Read the model definition and answer for the solid it produces. Units are mm, in the model's axes. A direction names the side the tool comes from. Coordinates: 2 decimals unless noted, no trailing zeros. Write each loop counter-clockwise with the first axis right and the second up, starting at its lowest first coordinate (ties: lowest second). Pieces come first, ordered by that corner, then holes. Notation, with made-up numbers: (-36, 47) -> (-25, 47) arc R14 ccw to (-25, 70) -> close; hole circle Ø10 at (24, 68.25). An arc over 180 degrees is marked (long way). One line per item, written item: value. Start each with the question number.
1. Given P1, Ø10, axis at x = 24, y = 45, coming from the -Z side; P2, Ø0.6, axis at y = 44, z = 1, coming from the +X side; P3, Ø1, axis at y = 37.5, z = 1, coming from the -X side; P4, Ø0.7, axis at y = 53.5, z = 0.5, coming from the +X side, each flat-ended and moving along its own axis, determine where each tip first touches the part or whether it passes through.
2. Find section A-A, the plane y = 35.5. Write down the section's boundary in (x, z).
3. Consider line 1 along X through (y, z) = (54.5, 1.95); line 2 along X through (y, z) = (43.5, 0.45); line 3 along Y through (x, z) = (15.5, 1.6). Determine where each line is inside the solid, lowest interval first.
4. For faces 1 (the flat face through (28.1, 57.08, 0.99)), 2 (the flat face through (41.827, 49.47, 0.986)), 3 (the flat face through (10.378, 39, 1)), determine the directions among +Z, -Z, +X, -X, +Y, -Y from which every point of the face is accessible in a straight line to the end or side of a thin tool.
5. Find section B-B, the plane x = 29. Write down the section's boundary in (y, z).
```python
from build123d import *

# Parameters (mm, degrees)
F1_DEPTH = 2


with BuildPart() as f1:
    # F0 (on Top) → F1 (new body)
    with BuildSketch(Plane.XY):
        Polygon((10.316424, 46.21381), (10.378422, 45.792866), (10.378422, 32.24406), (10.922515, 31.239605), (11.388969, 30.782871), (12.3236, 30.607224), (13.063584, 30.607224), (13.980744, 31.123197), (14.411193, 31.909108), (14.195969, 45.771692), (14.505405, 46.336659), (14.951889, 46.75483), (15.547823, 46.764082), (16.267732, 46.618171), (16.767925, 46.196714), (16.955901, 45.625031), (17.061751, 38.807264), (17.342532, 38.290832), (17.816337, 37.93142), (18.39029, 37.777532), (19.1046, 37.788622), (19.633163, 38.07852), (19.958686, 38.672859), (20.130083, 39.338022), (20.130083, 45.869723), (20.224372, 46.235643), (20.517316, 46.503272), (21.081642, 46.512033), (39.306525, 46.794985), (39.82532, 47.116615), (40.338621, 47.479954), (41.258305, 48.273247), (41.635639, 48.962181), (42.02386, 49.992487), (42.008081, 51.008835), (41.635639, 51.823597), (40.777957, 52.81793), (39.679653, 53.419479), (38.45059, 53.736179), (37.345576, 53.719023), (36.693033, 53.5032), (35.996381, 52.902289), (35.486977, 52.462892), (35.121937, 52.148019), (34.468539, 52.243274), (33.846248, 52.497253), (33.542935, 53.056076), (33.542935, 53.990863), (33.238664, 54.682236), (32.856002, 55.402562), (32.352884, 55.98584), (31.721991, 56.476444), (30.923305, 56.91389), (30.231845, 57.161622), (29.377455, 57.263315), (28.54972, 57.161622), (27.647492, 56.998174), (27.101057, 56.685288), (26.424225, 56.101473), (25.806281, 55.568452), (25.401196, 55.0007), (25.182293, 54.601029), (24.914882, 54.112791), (24.691492, 53.920102), (24.348679, 53.857998), (23.43077, 53.843747), (23.063278, 54.269789), (22.938367, 54.959297), (22.745963, 55.637598), (22.354444, 56.271017), (21.897662, 56.998174), (21.295404, 57.541236), (20.676884, 57.880004), (19.87285, 58.320378), (18.866845, 58.30476), (17.419982, 58.282296), (16.487831, 58.031149), (15.852839, 57.576239), (15.281766, 57.083648), (14.737288, 56.613998), (14.181019, 55.884421), (13.927415, 55.262856), (13.732859, 54.507815), (13.479641, 54.045492), (13.071425, 53.935507), (12.569794, 53.845812), (12.017341, 54.134376), (11.315221, 54.545794), (9.885113, 54.914299), (8.924496, 54.899385), (7.908149, 54.625553), (7.127685, 54.270785), (6.658861, 53.866391), (6.18615, 53.341925), (5.873267, 52.793737), (5.551593, 52.206428), (5.345334, 51.640082), (5.28802, 51.033568), (5.30319, 50.05647), (5.558579, 49.329612), (5.919253, 48.639685), (6.434358, 48.04251), (6.987177, 47.476605), (7.680411, 47.080936), (8.60151, 46.729587), (9.445827, 46.648875), (10.082705, 46.484766), align=None)
    extrude(amount=F1_DEPTH)


solid = f1.part
```
Answer block:
1. P1: stops at z = 0
1. P2: stops at x = 20.13
1. P3: stops at x = 10.38
1. P4: stops at x = 40.17
2. outline: (10.38, 0) -> (14.36, 0) -> (14.36, 2) -> (10.38, 2) -> close
3. line 1: x = 7.63 to 11.39, 13.73 to 23.02, 25.13 to 33.32
3. line 2: x = 10.38 to 14.23, 16.99 to 20.13
3. line 3: y = 46.76 to 57.27
4. face 1: +Z, -Z, +Y
4. face 2: +Z, -Z, +X, -Y
4. face 3: +Z, -Z, -X, -Y
5. outline: (46.63, 0) -> (57.22, 0) -> (57.22, 2) -> (46.63, 2) -> close
